Check sheet for the drawn part. Datum: minimum x, y, z corner. Units: mm. Give positions to 0.01 mm unless a question says otherwise; leave off trailing zeros. Order: outer loops, then holes, each group sorted by start corner. A loop starts at its lowest first (then second) coordinate and runs counter-clockwise, first axis right, second up.
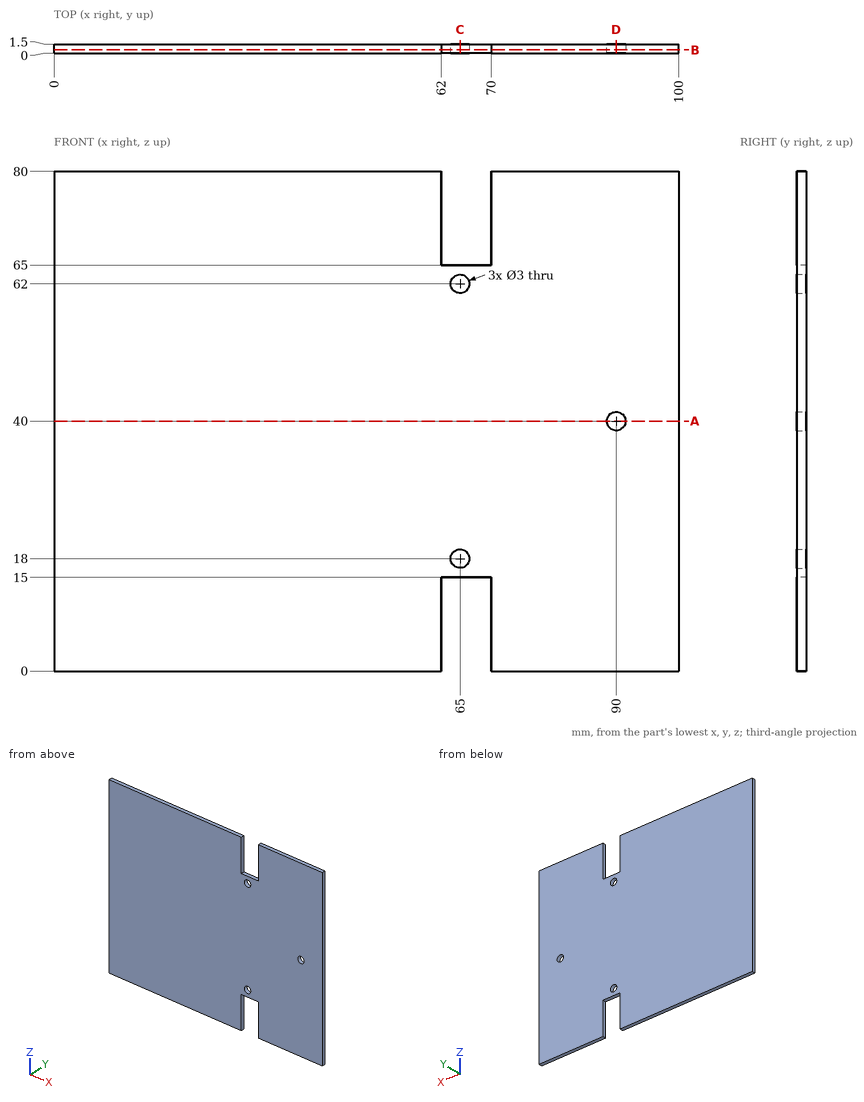
Q1. Material ranges on line 1 (Z direction, x = 65, y = 0.3); line 2 (X direction, y = 0.7, z = 40); line 3 (X direction, y = 1.2, z = 69), recorded low to high.
Q2. Sectioned sample at A-A, the plane z = 40. Record the cut outline in (x, y), plus the area to 4 significant figures.
Q3. Sectioned sample at C-C, the plane x = 65. Record the cut outline in (y, z), plus the area to 3 significant figures.
Q4. Sectioned sample at D-D, the plane x = 90. Record the cut outline in (y, z), plus the area to 4 significant figures.
Q5. Go/stop test with a flat-tipped pin: P1, Ø0.8, axis at x = 67, y = 0.5, coming from the +Z side. Record where the tip stops, or that it passes through.
Q6. Sectioned sample at B-B, the plane y = 0.55. Record the cut outline in (x, z), plus the area to 3 significant figures.
Filled in:
1. line 1: z = 15 to 16.5, 19.5 to 60.5, 63.5 to 65
1. line 2: x = 0 to 88.5, 91.5 to 100
1. line 3: x = 0 to 62, 70 to 100
2. outline: (0, 0) - (88.5, 0) - (88.5, 1.5) - (0, 1.5) - close; (91.5, 0) - (100, 0) - (100, 1.5) - (91.5, 1.5) - close
2. area: 145.5 mm2
3. outline: (0, 15) - (1.5, 15) - (1.5, 16.5) - (0, 16.5) - close; (0, 19.5) - (1.5, 19.5) - (1.5, 60.5) - (0, 60.5) - close; (0, 63.5) - (1.5, 63.5) - (1.5, 65) - (0, 65) - close
3. area: 66.0 mm2
4. outline: (0, 0) - (1.5, 0) - (1.5, 38.5) - (0, 38.5) - close; (0, 41.5) - (1.5, 41.5) - (1.5, 80) - (0, 80) - close
4. area: 115.5 mm2
5. P1: stops at z = 65
6. outline: (0, 0) - (62, 0) - (62, 15) - (70, 15) - (70, 0) - (100, 0) - (100, 80) - (70, 80) - (70, 65) - (62, 65) - (62, 80) - (0, 80) - close; hole circle Ø3 at (65, 18); hole circle Ø3 at (65, 62); hole circle Ø3 at (90, 40)
6. area: 7,740 mm2
